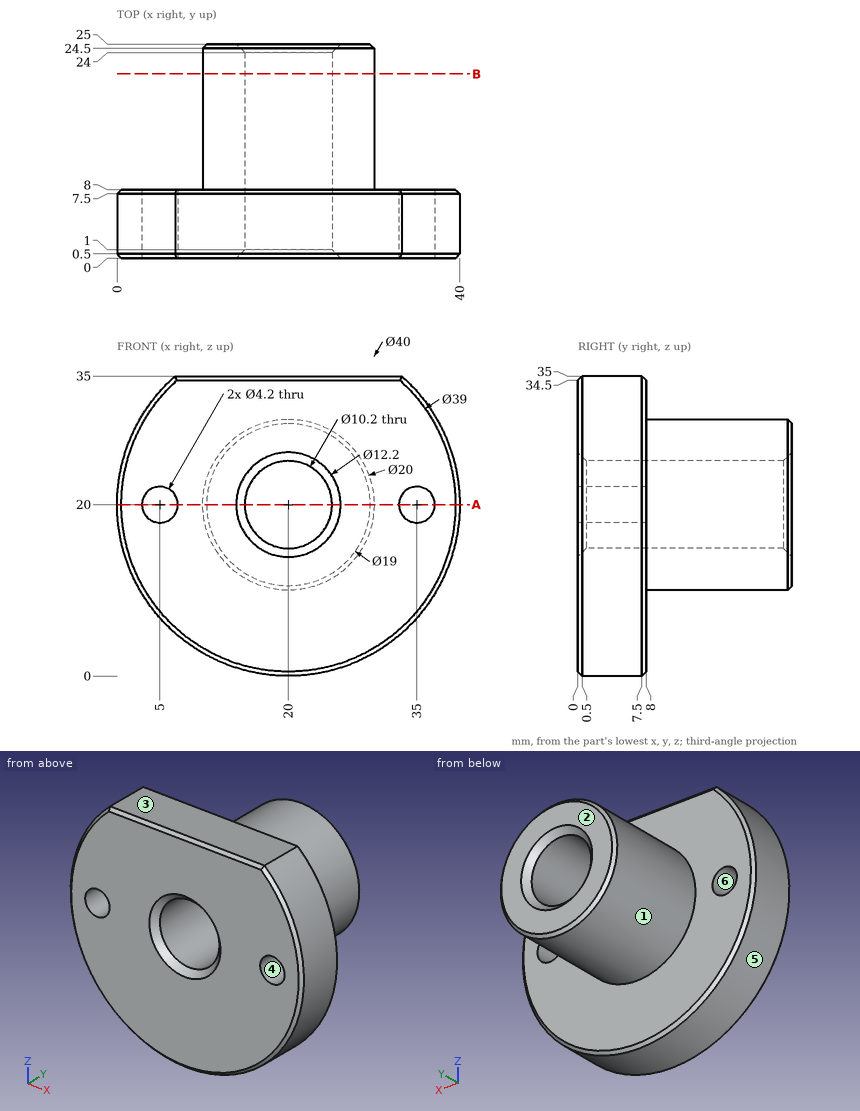
Part print with two shaded views. Sizes in mm from the minimum x, y, z corner. A direction names the side the tool comes from. Give positions to 0.01 mm unless a question says otherwise; leave off trailing zeros. Write each loop counter-clockwise with the first axis right and the second up, starting at its lowest first coordinate (ties: lowest second). Pieces come first, ordered by that corner, then holes.
1) Cut at B-B on y = 21.5. Write the cut outline in (x, z).
Resolved:
outline: circle Ø20 at (20, 20); hole circle Ø10.2 at (20, 20)
2) Which spindle directions (+Z, -Z, +X, -X, +Y, -Y) get a long thin tool onto all of the face, cutting with end or side? Do the marked faces 1 and 2. Say none if no direction does.
Resolved:
face 1: +Y
face 2: +Z, -Z, +X, -X, +Y
3) Cut at A-A on z = 20. State how many separate pieces and enclosed holes the cut face has, then the cut area to 3 significant figures.
Resolved:
separate pieces: 4
enclosed holes: 0
area: 335 mm2
4) Two-plate mould, pull along X, no slides. Class the marked faces 3, 4, 5 and 6: released by +X, released by -X, zero draft, split by the parting line, or undercut.
Resolved:
face 3: zero draft
face 4: undercut
face 5: split by the parting line
face 6: undercut
5) Probe L1, parallel to Z at x = 5, y = 4.5; L2, parallel to Z at x = 17.5, y = 12; L3, parallel to Y at x = 30.5, z = 7. List the from-to ranges inside material, lowest first.
Resolved:
L1: z = 6.77 to 17.9, 22.1 to 33.23
L2: z = 10.32 to 15.55, 24.45 to 29.68
L3: y = 0 to 8
6) Pin check, flat tips, straight feed: pin 1 (1 mm diameter, centred on x = 18, y = 18.5, fed in from +Z); pin 2 (10 mm diameter, centred on y = 14, z = 13.5, fed in from -X); pin 3 (3 mm diameter, centred on y = 21.5, z = 19.5, fed in from -X). Stop position of each tip, or through.
Resolved:
pin 1: stops at z = 29.89
pin 2: stops at x = 10.11
pin 3: stops at x = 10
